from build123d import *

# Parameters (mm, degrees)
F1_DEPTH = 25


with BuildPart() as f1:
    # F0 (on Top) → F1 (new body)
    with BuildSketch(Plane.XY):
        with BuildLine():
            ThreePointArc((-42, 0), (0, 42), (42, 0))
            Line((42, 0), (62.329768, 0))
            Line((62.329768, 0), (73, 0))
            Line((73, 0), (182, 0))
            Line((182, 0), (182, 38))
            Line((182, 38), (62.329768, 38))
            ThreePointArc((62.329768, 38), (-19.734829, 70.281836), (-73, 0))
            Line((-73, 0), (-42, 0))
        make_face()
    extrude(amount=F1_DEPTH)


solid = f1.part
For this review, take the finished solid that the model builds, in its own axes (mm). A direction names the side the tool comes from. Give positions to 0.01 mm unless a question says otherwise; leave off trailing zeros. Loops run counter-clockwise (first coordinate to the right, second up) from the corner with the lowest first, then second, coordinate; pieces in that order, holes last. Notation, with made-up numbers: (-40, -23.5) - (16, -23.5) arc R30 ccw to (16, 15.5) - close; hole circle Ø3 at (67.25, 3.5). An arc over 180 degrees is marked (long way). Write each question's results on one line, items separated by ' | '.
(1) For faces 1 (the flat face through (111, 0, 12)), 2 (the flat face through (123, 38, 12)), list the 3-axis set-ups (+Z, -Z, +X, -X, +Y, -Y) from which the entire face can be reached by the end or side of a thin tool; tool diameter is ignored.
Conclusion:
face 1: +Z, -Z, +X, -X, -Y | face 2: +Z, -Z, +X, +Y
(2) Take a section at B-B (z = 8.25). Give the boundary of the cut face in (x, y).
Conclusion:
outline: (-73, 0) - (-42, 0) arc R42 cw to (42, 0) - (182, 0) - (182, 38) - (62.33, 38) arc R73 ccw to start
(3) Take a section at C-C (x = 0). Give the boundary of the cut face in (y, z), then the cut area to 3 significant figures.
Conclusion:
outline: (42, 0) - (73, 0) - (73, 25) - (42, 25) - close | area: 775 mm^2
(4) For line 1 along X through (y, z) = (8, 22.5); line 2 along Y through (x, z) = (129.5, 8.5); line 3 along X through (y, z) = (29.5, 15.25), list the stretches that pass through material, from the lowest coordinate up.
Conclusion:
line 1: -72.56 to -41.23, 41.23 to 182 | line 2: 0 to 38 | line 3: -66.77 to -29.9, 29.9 to 182
(5) Take a section at D-D (y = 48). Give the boundary of the cut face in (x, z), then the cut area to 3 significant figures.
Conclusion:
outline: (-55, 0) - (55, 0) - (55, 25) - (-55, 25) - close | area: 2,750 mm^2
(6) For pin 1 Ø6 at (x, z) = (71.5, 16.5) entering from +Y; pin 2 Ø1 at (x, z) = (9.5, 11) entering from +Y; pin 3 Ø1 at (x, z) = (11, 10.5) entering from +Y, all flat-tipped, find the tip position at first contact; note any pin that passes through.
Conclusion:
pin 1: y = 38 | pin 2: y = 72.44 | pin 3: y = 72.24
(7) Draft analysis for pull direction X (two halves, no side actions). For faces 3 (the flat face through (53, 29, 25)), 4 (the flat face through (182, 19, 12)), 5 (the cylindrical face through (-0.92, 41.99, 12.32)), state which applies: +X half, -X half, draft (parallel to the pull), parting line (faces both ways), or undercut.
Conclusion:
face 3: draft | face 4: +X half | face 5: undercut
(8) Take a section at A-A (y = 6). Give the boundary of the cut face in (x, z).
Conclusion:
outline: (-72.75, 0) - (-41.57, 0) - (-41.57, 25) - (-72.75, 25) - close; (41.57, 0) - (182, 0) - (182, 25) - (41.57, 25) - close
